from build123d import *

# Parameters (mm, degrees)
SKETCH1_W            = 150
SKETCH1_H            = 42
BOSS_EXTRUDE1_DEPTH  = 3.2
SKETCH2_W            = 162
SKETCH2_H            = 52
BOSS_EXTRUDE2_DEPTH  = 6
SKETCH3_W            = 6
SKETCH3_H            = 52
BOSS_EXTRUDE3_DEPTH  = 176
BOSS_EXTRUDE4_REACH  = 238.618
SKETCH5_W            = 52
SKETCH5_H            = 6
BOSS_EXTRUDE5_START  = 100
SKETCH1_2_W          = 150
SKETCH1_2_H          = 42
BOSS_EXTRUDE5_DEPTH  = 3.2
SKETCH6_W            = 150
SKETCH6_H            = 6
BOSS_EXTRUDE6_DEPTH  = 70
CUT_EXTRUDE1_REACH   = 142.645
SKETCH7_W            = 10
SKETCH7_H            = 40
SKETCH7_R            = 3
SKETCH7_3_W          = 6
SKETCH7_3_H          = 40
BOSS_EXTRUDE7_DEPTH  = 54
SKETCH8_W            = 162
SKETCH8_H            = 10
BOSS_EXTRUDE8_DEPTH  = 3.2
SKETCH9_W            = 150
SKETCH9_H            = 42
CUT_EXTRUDE2_DEPTH   = 3.2
CUT_EXTRUDE3_DEPTH   = 3.2
BOSS_EXTRUDE9_DEPTH  = 3.2
SKETCH12_W           = 3.2
SKETCH12_H           = 10
BOSS_EXTRUDE10_DEPTH = 6
CUT_EXTRUDE4_REACH   = 236.897
SKETCH13_R           = 4
CUT_EXTRUDE5_REACH   = 201.894
SKETCH14_R           = 1
SKETCH16_W           = 6
SKETCH16_H           = 172
BOSS_EXTRUDE11_DEPTH = 3.2
SKETCH17_W           = 162
SKETCH17_H           = 58.4
SKETCH17_W_2         = 150
SKETCH17_H_2         = 52
BOSS_EXTRUDE12_DEPTH = 6
SKETCH15_R           = 1
BOSS_EXTRUDE14_DEPTH = 3.2
FILLET1_R            = 2
FILLET1_OF_MIRROR4_R = 2


with BuildPart() as part:
    # Sketch1 → Boss-Extrude1 (new body)
    with BuildSketch(Plane(origin=(0, 0, 0), x_dir=(1, 0, 0), z_dir=(0, 1, 0))):
        Rectangle(SKETCH1_W, SKETCH1_H)
    extrude(amount=BOSS_EXTRUDE1_DEPTH)

    # Sketch2 → Boss-Extrude2 (add)
    with BuildSketch(Plane.XZ):
        Rectangle(SKETCH2_W, SKETCH2_H)
    extrude(amount=BOSS_EXTRUDE2_DEPTH)

    # Sketch3 → Boss-Extrude3 (add)
    with BuildSketch(Plane(origin=(0, 0, 0), x_dir=(1, 0, 0), z_dir=(0, 1, 0))):
        with Locations((78, 0)):
            Rectangle(SKETCH3_W, SKETCH3_H)
        with Locations((-78, 0)):
            Rectangle(SKETCH3_W, SKETCH3_H)
    extrude(amount=BOSS_EXTRUDE3_DEPTH)

    # Sketch5 → Boss-Extrude4 (add, up to next)
    with BuildSketch(Plane.ZY.offset(-75), mode=Mode.PRIVATE) as boss_extrude4_sk1:
        with Locations((0, 103)):
            Rectangle(SKETCH5_W, SKETCH5_H)
    boss_extrude4_tool1 = extrude(boss_extrude4_sk1.sketch, amount=BOSS_EXTRUDE4_REACH, mode=Mode.PRIVATE) - part.part
    add(boss_extrude4_tool1.solids().sort_by_distance((75, 103, 0))[0])

    # Sketch1<2> → Boss-Extrude5 (add)
    with BuildSketch(Plane(origin=(0, 0, 0), x_dir=(1, 0, 0), z_dir=(0, 1, 0)).offset(BOSS_EXTRUDE5_START)):
        Rectangle(SKETCH1_2_W, SKETCH1_2_H)
    extrude(amount=-BOSS_EXTRUDE5_DEPTH)

    # Sketch6 → Boss-Extrude6 (add)
    with BuildSketch(Plane(origin=(0, 106, 0), x_dir=(1, 0, 0), z_dir=(0, 1, 0))):
        with Locations((0, -23)):
            Rectangle(SKETCH6_W, SKETCH6_H)
        with Locations((0, 23)):
            Rectangle(SKETCH6_W, SKETCH6_H)
    extrude(amount=BOSS_EXTRUDE6_DEPTH)

    # Sketch7 → Cut-Extrude1 (cut, up to next)
    with BuildSketch(Plane(origin=(0, 106, 0), x_dir=(1, 0, 0), z_dir=(0, 1, 0)), mode=Mode.PRIVATE) as cut_extrude1_sk1:
        with Locations((70, 0)):
            Rectangle(SKETCH7_W, SKETCH7_H)
        with Locations((70, -15)):
            Circle(SKETCH7_R, mode=Mode.SUBTRACT)
        with Locations((70, 15)):
            Circle(SKETCH7_R, mode=Mode.SUBTRACT)
    cut_extrude1_tool1 = extrude(cut_extrude1_sk1.sketch, amount=-CUT_EXTRUDE1_REACH, mode=Mode.PRIVATE) & part.part
    # Sketch7 → Cut-Extrude1 (cut, up to next)
    with BuildSketch(Plane(origin=(0, 106, 0), x_dir=(1, 0, 0), z_dir=(0, 1, 0)), mode=Mode.PRIVATE) as cut_extrude1_sk2:
        with Locations((70, -15)):
            Circle(SKETCH7_R)
    cut_extrude1_tool2 = extrude(cut_extrude1_sk2.sketch, amount=-CUT_EXTRUDE1_REACH, mode=Mode.PRIVATE) & part.part
    # Sketch7 → Cut-Extrude1 (cut, up to next)
    with BuildSketch(Plane(origin=(0, 106, 0), x_dir=(1, 0, 0), z_dir=(0, 1, 0)), mode=Mode.PRIVATE) as cut_extrude1_sk3:
        with Locations((70, 15)):
            Circle(SKETCH7_R)
    cut_extrude1_tool3 = extrude(cut_extrude1_sk3.sketch, amount=-CUT_EXTRUDE1_REACH, mode=Mode.PRIVATE) & part.part
    add(cut_extrude1_tool1.solids().sort_by_distance((70, 106, 0))[0], mode=Mode.SUBTRACT)
    add(cut_extrude1_tool2.solids().sort_by_distance((70, 106, 15))[0], mode=Mode.SUBTRACT)
    add(cut_extrude1_tool3.solids().sort_by_distance((70, 106, -15))[0], mode=Mode.SUBTRACT)

    # Sketch7<3> → Boss-Extrude7 (add)
    with BuildSketch(Plane(origin=(0, 106, 0), x_dir=(1, 0, 0), z_dir=(0, 1, 0))):
        with Locations((62, 0)):
            Rectangle(SKETCH7_3_W, SKETCH7_3_H)
    extrude(amount=BOSS_EXTRUDE7_DEPTH)

    # Sketch8 → Boss-Extrude8 (add)
    with BuildSketch(Plane(origin=(0, 0, -26), x_dir=(-1, 0, 0), z_dir=(0, 0, -1))):
        with Locations((0, -1)):
            Rectangle(SKETCH8_W, SKETCH8_H)
    boss_extrude8 = extrude(amount=BOSS_EXTRUDE8_DEPTH)

    # Mirror1: Boss-Extrude8 across plane
    add(boss_extrude8.mirror(Plane.XY))

    # Sketch9 → Cut-Extrude2 (cut)
    with BuildSketch(Plane(origin=(0, 3.2, 0), x_dir=(1, 0, 0), z_dir=(0, 1, 0))):
        Rectangle(SKETCH9_W, SKETCH9_H)
    extrude(amount=-CUT_EXTRUDE2_DEPTH, mode=Mode.SUBTRACT)

    # Sketch10 → Cut-Extrude3 (cut)
    with BuildSketch(Plane.XZ.offset(-96.8)):
        Polygon((-75, -21), (75, -21), (75, -20), (65, -20), (65, 20), (75, 20), (75, 21), (-75, 21), align=None)
    extrude(amount=-CUT_EXTRUDE3_DEPTH, mode=Mode.SUBTRACT)

    # Sketch11 → Boss-Extrude9 (add)
    with BuildSketch(Plane.ZY.offset(-75)):
        Polygon((10, 93.5), (-21, 93.5), (-21, 0), (21, 0), (21, 100), (10, 100), align=None)
    boss_extrude9 = extrude(amount=BOSS_EXTRUDE9_DEPTH)

    # Mirror2: Boss-Extrude9 across plane
    add(boss_extrude9.mirror(Plane(origin=(0, 0, 0), x_dir=(0, 0, 1), z_dir=(1, 0, 0))))

    # Sketch12 → Boss-Extrude10 (add)
    with BuildSketch(Plane(origin=(0, 100, 0), x_dir=(1, 0, 0), z_dir=(0, 1, 0))):
        with Locations((73.4, -15)):
            Rectangle(SKETCH12_W, SKETCH12_H)
    extrude(amount=BOSS_EXTRUDE10_DEPTH)

    # Sketch13 → Cut-Extrude4 (cut, up to next)
    with BuildSketch(Plane.ZY.offset(-71.8), mode=Mode.PRIVATE) as cut_extrude4_sk1:
        with Locations((0, 20)):
            Circle(SKETCH13_R)
    cut_extrude4_tool1 = extrude(cut_extrude4_sk1.sketch, amount=-CUT_EXTRUDE4_REACH, mode=Mode.PRIVATE) & part.part
    add(cut_extrude4_tool1.solids().sort_by_distance((71.8, 20, 0))[0], mode=Mode.SUBTRACT)

    # Sketch14 → Cut-Extrude5 (cut, up to next)
    with BuildSketch(Plane.XY.offset(-20), mode=Mode.PRIVATE) as cut_extrude5_sk1:
        with Locations((62, 103)):
            Circle(SKETCH14_R)
    cut_extrude5_tool1 = extrude(cut_extrude5_sk1.sketch, amount=-CUT_EXTRUDE5_REACH, mode=Mode.PRIVATE) & part.part
    # Sketch14 → Cut-Extrude5 (cut, up to next)
    with BuildSketch(Plane.XY.offset(-20), mode=Mode.PRIVATE) as cut_extrude5_sk2:
        with Locations((62, 109)):
            Circle(SKETCH14_R)
    cut_extrude5_tool2 = extrude(cut_extrude5_sk2.sketch, amount=-CUT_EXTRUDE5_REACH, mode=Mode.PRIVATE) & part.part
    # Sketch14 → Cut-Extrude5 (cut, up to next)
    with BuildSketch(Plane.XY.offset(-20), mode=Mode.PRIVATE) as cut_extrude5_sk3:
        with Locations((62, 115)):
            Circle(SKETCH14_R)
    cut_extrude5_tool3 = extrude(cut_extrude5_sk3.sketch, amount=-CUT_EXTRUDE5_REACH, mode=Mode.PRIVATE) & part.part
    add(cut_extrude5_tool1.solids().sort_by_distance((62, 103, -20))[0], mode=Mode.SUBTRACT)
    add(cut_extrude5_tool2.solids().sort_by_distance((62, 109, -20))[0], mode=Mode.SUBTRACT)
    add(cut_extrude5_tool3.solids().sort_by_distance((62, 115, -20))[0], mode=Mode.SUBTRACT)

    # Sketch16 → Boss-Extrude11 (add)
    with BuildSketch(Plane(origin=(0, 0, -26), x_dir=(-1, 0, 0), z_dir=(0, 0, -1))):
        with Locations((78, 90)):
            Rectangle(SKETCH16_W, SKETCH16_H)
        with Locations((-78, 90)):
            Rectangle(SKETCH16_W, SKETCH16_H)
    boss_extrude11 = extrude(amount=BOSS_EXTRUDE11_DEPTH)

    # Mirror3: Boss-Extrude11 across plane
    add(boss_extrude11.mirror(Plane.XY))

    # Sketch17 → Boss-Extrude12 (add)
    with BuildSketch(Plane.XZ.offset(6)):
        Rectangle(SKETCH17_W, SKETCH17_H)
        Rectangle(SKETCH17_W_2, SKETCH17_H_2, mode=Mode.SUBTRACT)
    extrude(amount=BOSS_EXTRUDE12_DEPTH)

    # Sketch15 → Boss-Extrude14 (add)
    with BuildSketch(Plane(origin=(0, 0, -26), x_dir=(-1, 0, 0), z_dir=(0, 0, -1))):
        with BuildLine():
            ThreePointArc((-62, 121.5), (-50.407976881, 113.677071733), (-53.325324214, 100))
            Line((-53.325324214, 100), (-46, 100))
            Line((-46, 100), (-46, 121.5))
            Line((-46, 121.5), (-62, 121.5))
        make_face()
        with BuildLine():
            ThreePointArc((-62, 121.5), (-73.592023119, 113.677071733), (-70.674675786, 100))
            Line((-70.674675786, 100), (-53.325324214, 100))
            ThreePointArc((-53.325324214, 100), (-50.407976881, 113.677071733), (-62, 121.5))
        make_face()
        with Locations(Location((-62, 103, 0), (0, 0, 180))):
            Circle(SKETCH15_R, mode=Mode.SUBTRACT)
        with Locations(Location((-62, 109, 0), (0, 0, 180))):
            Circle(SKETCH15_R, mode=Mode.SUBTRACT)
        with Locations(Location((-62, 115, 0), (0, 0, 180))):
            Circle(SKETCH15_R, mode=Mode.SUBTRACT)
    boss_extrude14 = extrude(amount=BOSS_EXTRUDE14_DEPTH)

    # Fillet1
    fillet1_edges = [part.edges().sort_by_distance(p)[0] for p in [
        (46, 121.5, -27.6),
        (46, 100, -27.6),
    ]]
    fillet(fillet1_edges, radius=FILLET1_R)

    # Mirror4: Boss-Extrude14 across plane
    add(boss_extrude14.mirror(Plane.XY))

    # Fillet1 of Mirror4
    fillet1_of_mirror4_edges = [part.edges().sort_by_distance(p)[0] for p in [
        (46, 121.5, 27.6),
        (46, 100, 27.6),
    ]]
    fillet(fillet1_of_mirror4_edges, radius=FILLET1_OF_MIRROR4_R)


solid = part.part
Work out the finished part from the listing and answer in its coordinate system (mm). A direction names the side the tool comes from. Coordinates: 2 decimals unless noted, no trailing zeros. Loops run counter-clockwise (first coordinate to the right, second up) from the corner with the lowest first, then second, coordinate; pieces in that order, holes last. Notation, with made-up numbers: M 49.25,53 L 97.25,53 A23 cw 97.25,65 Z; hole C 66,42 d8. An arc over 180 degrees is marked long. Answer in a Markdown table with one row per item. Add a question column.
1. The mould has two halves that part along Y. Classify faces 6 (the flat face through (-7, 106, 0)), 7 (the flat face through (-1, 0, 0)), 8 (the flat face through (1, -6, 0)): pulls with the +Y half, pulls with the -Y half, needs draft (parallel to the pull), parting line crosses it, or undercut.
2. Flat-ended cylindrical pins translate along their axes: P1, Ø1.6, axis at x = -72.5, y = 53.5, coming from the -Z side; P2, Ø1, axis at x = 37.5, y = 130.5, coming from the -Z side; P3, Ø3.5, axis at x = 5, z = 28, coming from the +Y side. Find the tip coordinate at first contact, or state that the pin passes through.
3. Find section B-B, the plane y = 20. Write down the section's boundary in (x, z).
4. Find section C-C, the plane z = 0. Write down the section's boundary in (x, y).
5. Consider L1, parallel to X at y = 109, z = -26.75; L2, parallel to Y at x = 62, z = 28; L3, parallel to X at y = 126.5, z = 11. Determine where each line is inside the solid, lowest interval first.
6. A tool of negligible diameter and unlimited length cuts with its end or side. For faces 1 (the flat face through (60, 111, -29.2)), 2 (the flat face through (1, 2, 26)), 3 (the flat face through (-75, 141, 0)), 4 (the flat face through (-1, -9, -26)), 5 (the cylindrical face through (73.5, 113.9, -27.6)), from which of +Z, -Z, +X, -X, +Y, -Y can it reach the whole face along a straight path? Write none if from no direction.
7. Find section D-D, the plane x = -66. Write down the section's boundary in (y, z).
8. Find section A-A, the plane y = 90. Write down the section's boundary in (x, z), then the cut area to 3 significant figures.
Reported:
| question | item | result |
|---|---|---|
| 1 | face 6 | pulls with the +Y half |
| 1 | face 7 | undercut |
| 1 | face 8 | pulls with the -Y half |
| 2 | P1 | stops at z = -21 |
| 2 | P2 | stops at z = -26 |
| 2 | P3 | stops at y = 4 |
| 3 | outline | M -81,-29.2 L -75,-29.2 L -75,-21 L -71.8,-21 L -71.8,21 L -75,21 L -75,29.2 L -81,29.2 Z; M 71.8,-21 L 75,-21 L 75,-29.2 L 81,-29.2 L 81,-4 L 71.8,-4 Z; M 71.8,4 L 81,4 L 81,29.2 L 75,29.2 L 75,21 L 71.8,21 Z |
| 4 | outline | M -81,-12 L -75,-12 L -75,-6 L 75,-6 L 75,-12 L 81,-12 L 81,16 L 71.8,16 L 71.8,0 L -71.8,0 L -71.8,93.5 L -75,93.5 L -75,100 L 65,100 L 65,160 L 59,160 L 59,106 L -75,106 L -75,176 L -81,176 Z; M 71.8,24 L 81,24 L 81,176 L 75,176 L 75,93.5 L 71.8,93.5 Z |
| 5 | L1 | x = -81 to -75, 46 to 61, 63 to 74.5, 75 to 81 |
| 5 | L2 | y = -12 to 4, 100 to 102, 104 to 108, 110 to 114, 116 to 121.5 |
| 5 | L3 | x = -81 to -75, 59 to 65, 75 to 81 |
| 6 | face 1 | -Z, +X, -X, +Y, -Y |
| 6 | face 2 | none |
| 6 | face 3 | +Y |
| 6 | face 4 | -Y |
| 6 | face 5 | -Z |
| 7 | outline | M -12,-29.2 L 4,-29.2 L 4,-26 L 0,-26 L 0,26 L 4,26 L 4,29.2 L -12,29.2 L -12,26 L -6,26 L -6,-26 L -12,-26 Z; M 100,-26 L 176,-26 L 176,-20 L 106,-20 L 106,20 L 176,20 L 176,26 L 100,26 Z |
| 8 | outline | M -81,-29.2 L -75,-29.2 L -75,-21 L -71.8,-21 L -71.8,21 L -75,21 L -75,29.2 L -81,29.2 Z; M 71.8,-21 L 75,-21 L 75,-29.2 L 81,-29.2 L 81,29.2 L 75,29.2 L 75,21 L 71.8,21 Z |
| 8 | area | 970 mm^2 |
